For this review, use the dimensioned drawing (mm, ordinates from the lowest corner) and the shaded views. A direction names the side the tool comes from. Coordinates: 2 decimals unless noted, no trailing zeros. Write each loop counter-clockwise with the first axis right and the second up, starting at its lowest first coordinate (ties: lowest second). Pieces come first, ordered by that corner, then holes. Notation, with made-up numbers: (-32, 43.5) - (6, 43.5) arc R23 ccw to (6, 78.5) - close; hole circle Ø11 at (59, 86.25). An arc over 180 degrees is marked (long way). Put each result on its own line as item: value.
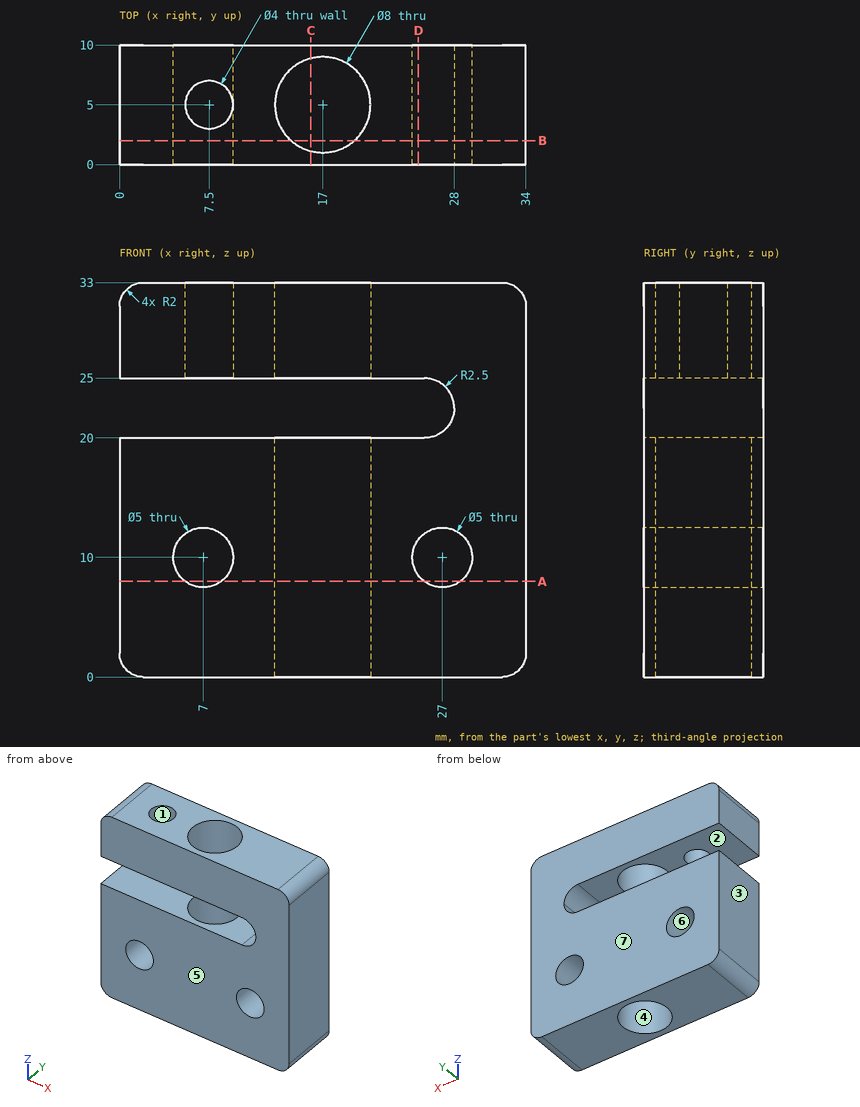
1. Consider section C-C on x = 16. State the section outline as (y, z) points.
Determined:
outline: (0, 0) - (1.13, 0) - (1.13, 20) - (0, 20) - close; (0, 25) - (1.13, 25) - (1.13, 33) - (0, 33) - close; (8.87, 0) - (10, 0) - (10, 20) - (8.87, 20) - close; (8.87, 25) - (10, 25) - (10, 33) - (8.87, 33) - close
2. Consider section B-B on y = 2. Give the number of separate pieces and of enclosed holes in the cut face, plus the area to 3 significant figures.
Determined:
separate pieces: 3
enclosed holes: 2
area: 794 mm^2
3. Machinability: for the marked faces 1, 2 and 3, which of the approach directions +Z, -Z, +X, -X, +Y, -Y give a long, thin tool a straight path to every point of the face, cutting with its end or side? Answer none if there is none.
Determined:
face 1: +Z
face 2: -X, +Y, -Y
face 3: +Z, -Z, -X, +Y, -Y
4. Consider section D-D on x = 25. State the section outline as (y, z) points, plus the area to 3 significant figures.
Determined:
outline: (0, 0) - (10, 0) - (10, 8.5) - (0, 8.5) - close; (0, 11.5) - (10, 11.5) - (10, 20) - (0, 20) - close; (0, 25) - (10, 25) - (10, 33) - (0, 33) - close
area: 250 mm^2
5. For pin 1 Ø6 at (y, z) = (3.5, 22) entering from -X; pin 2 Ø3 at (y, z) = (4.5, 22.5) entering from -X, all flat-tipped, find the tip position at first contact; note any pin that passes through.
Determined:
pin 1: stops at x = 0
pin 2: stops at x = 27.5
6. Consider section A-A on z = 8. State the section outline as (x, y) points.
Determined:
outline: (0, 0) - (5.5, 0) - (5.5, 10) - (0, 10) - close; (8.5, 0) - (25.5, 0) - (25.5, 10) - (8.5, 10) - close; (28.5, 0) - (34, 0) - (34, 10) - (28.5, 10) - close; hole circle Ø8 at (17, 5)
7. The part is to be moulded in two halves that separate along Y. For the marked faces 4, 5, 6 and 7, say which applies: +Y half, -Y half, draft (parallel to the pull), parting line (faces both ways), or undercut.
Determined:
face 4: undercut
face 5: -Y half
face 6: draft
face 7: +Y half
8. To check wall thickness, follow probe 1 along X at (y, z) = (3.5, 10); probe 2 along Y at (x, z) = (17, 31.5); probe 3 along Z at (x, y) = (22.5, 2). State the ranges of each line that lie inside material, in increasing order.
Determined:
probe 1: x = 0 to 4.5, 9.5 to 13.29, 20.71 to 24.5, 29.5 to 34
probe 2: y = 0 to 1, 9 to 10
probe 3: z = 0 to 20, 25 to 33
